Check sheet for the drawn part. Datum: minimum x, y, z corner. Units: mm. A direction names the side the tool comes from. Give positions to 0.01 mm unless a question says otherwise; leave off trailing zeros. Write each loop counter-clockwise with the first axis right and the second up, starting at its lowest first coordinate (ties: lowest second). Pieces come first, ordered by that corner, then holes. Notation, with made-up numbers: (7, 6.25) -> (30, 6.25) arc R12 cw to (30, 24.25) -> close; hole circle Ø1 at (11, -19). An arc over 180 degrees is marked (long way). Write item = value, one per line. Start each with the question number.
1. Cross-section at A-A, the plane y = 127. Record the cut outline in (x, z).
2. Cross-section at D-D, the plane z = 17.5. Record the cut outline in (x, y), plus the area to 3 significant figures.
3. Cross-section at C-C, the plane x = 11.75. Record the cut outline in (y, z).
4. Thickness scan on line 1 along Z through (x, y) = (3.5, 127); line 2 along Z through (x, y) = (22, 100.5). Record the ranges inside material, lowest first.
5. Depth check by flat-ended pin: P1, Ø8, axis at y = 126, z = 29.5, coming from the +X side; P2, Ø3, axis at x = 13, y = 54, coming from the +Z side; P3, Ø1.9, axis at x = 14, z = 4, coming from the -Y side. Enter the tip coordinate at first touch or a pass-through.
6. Cross-section at B-B, the plane y = 56. Record the cut outline in (x, z).
7. Set-up check for the marked faces 1 and 2: record each of +Z, -Z, +X, -X, +Y, -Y from which the full face is reachable in a straight line by a thin tool's end or side.
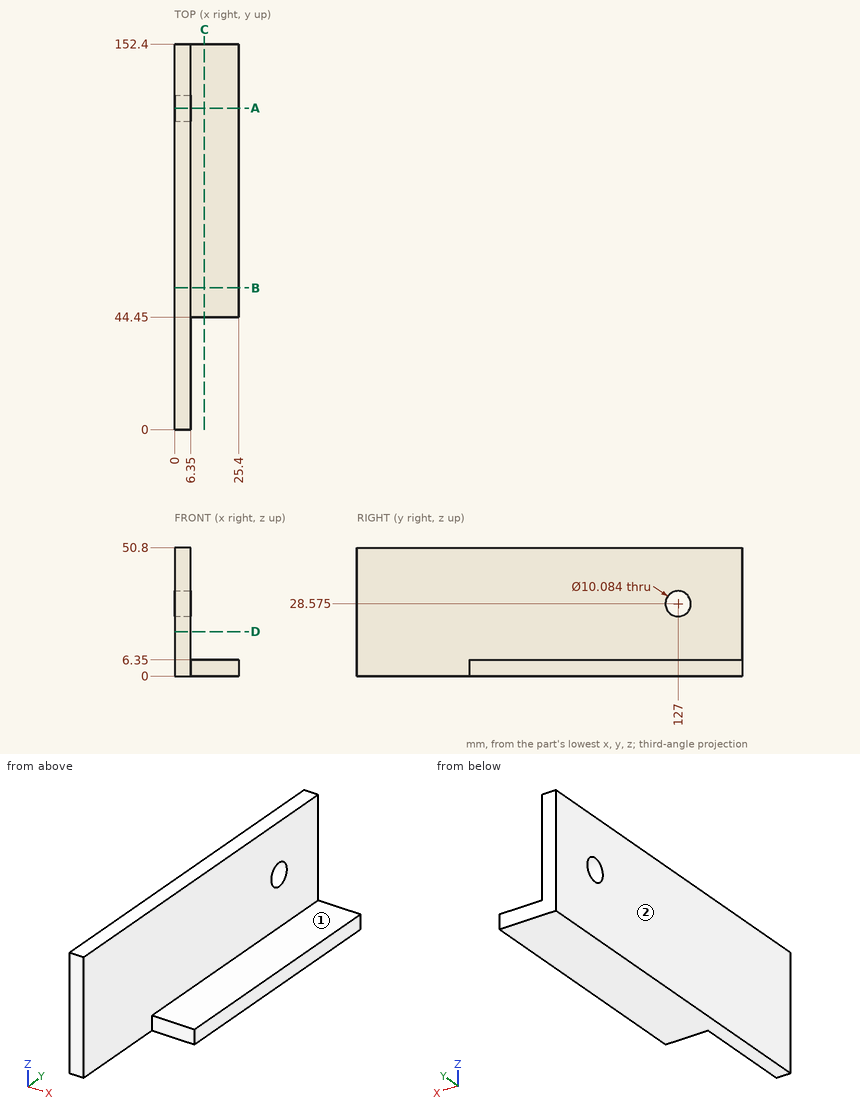
Answers:
q1.outline = (0, 0) -> (25.4, 0) -> (25.4, 6.35) -> (6.35, 6.35) -> (6.35, 23.53) -> (0, 23.53) -> close; (0, 33.62) -> (6.35, 33.62) -> (6.35, 50.8) -> (0, 50.8) -> close
q2.outline = (0, 0) -> (6.35, 0) -> (6.35, 152.4) -> (0, 152.4) -> close
q2.area = 968 mm^2
q3.outline = (44.45, 0) -> (152.4, 0) -> (152.4, 6.35) -> (44.45, 6.35) -> close
q4.line_1 = 0 to 23.53, 33.62 to 50.8
q4.line_2 = 0 to 6.35
q5.P1 = 6.35
q5.P2 = 6.35
q5.P3 = 44.45
q6.outline = (0, 0) -> (25.4, 0) -> (25.4, 6.35) -> (6.35, 6.35) -> (6.35, 50.8) -> (0, 50.8) -> close
q7.face_1 = +Z, +X, +Y, -Y
q7.face_2 = +Z, -Z, -X, +Y, -Y
